For this review, use the dimensioned drawing (mm, ordinates from the lowest corner) and the shaded views. A direction names the side the tool comes from. Coordinates: 2 decimals unless noted, no trailing zeros. Order: outer loops, then holes, each group sorted by start corner. A loop starts at its lowest first (then second) coordinate and runs counter-clockwise, first axis right, second up. Notation, with made-up numbers: M 78.5,56.25 L 127.5,56.25 A17 ccw 127.5,67.25 Z; hole C -5,50.5 d5. An arc over 180 degrees is marked long. Answer in a Markdown table with one row per item.
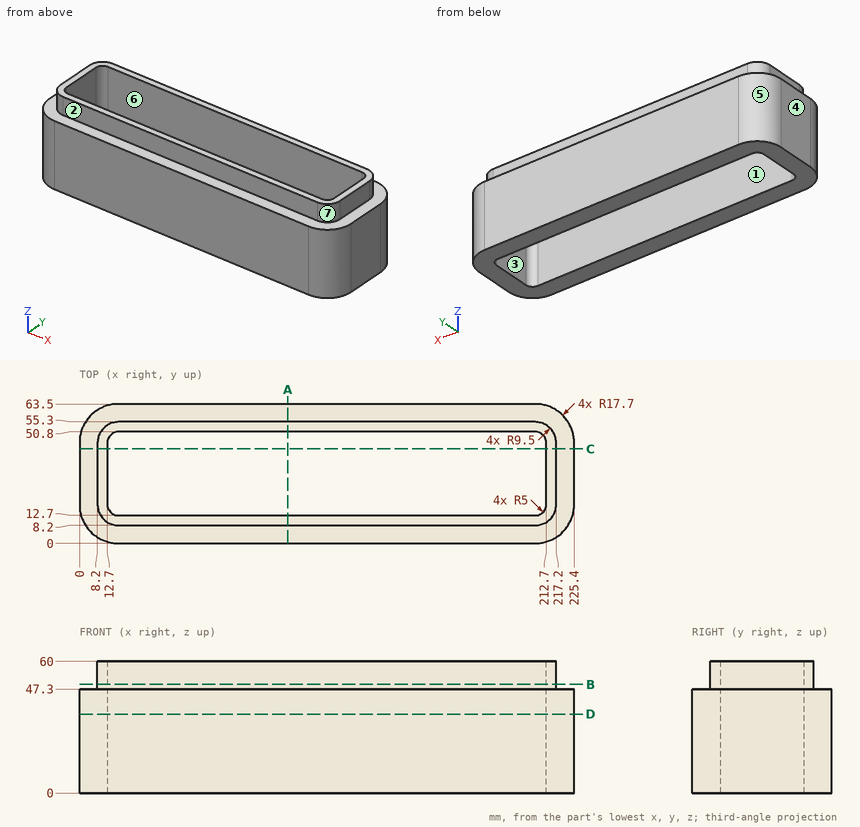
(1) Take a section at D-D (z = 36). Write out the cut boundary in (x, y), then the cut area to 3 significant figures.
Report:
| item | result |
|---|---|
| outline | M 0,17.7 A17.7 ccw 17.7,0 L 207.7,0 A17.7 ccw 225.4,17.7 L 225.4,45.8 A17.7 ccw 207.7,63.5 L 17.7,63.5 A17.7 ccw 0,45.8 Z; hole M 12.7,17.7 A5 ccw 17.7,12.7 L 207.7,12.7 A5 ccw 212.7,17.7 L 212.7,45.8 A5 ccw 207.7,50.8 L 17.7,50.8 A5 ccw 12.7,45.8 Z |
| area | 6,450 mm^2 |
(2) Take a section at B-B (z = 49.5). Write out the cut boundary in (x, y).
Report:
| item | result |
|---|---|
| outline | M 8.2,17.7 A9.5 ccw 17.7,8.2 L 207.7,8.2 A9.5 ccw 217.2,17.7 L 217.2,45.8 A9.5 ccw 207.7,55.3 L 17.7,55.3 A9.5 ccw 8.2,45.8 Z; hole M 12.7,17.7 A5 ccw 17.7,12.7 L 207.7,12.7 A5 ccw 212.7,17.7 L 212.7,45.8 A5 ccw 207.7,50.8 L 17.7,50.8 A5 ccw 12.7,45.8 Z |
(3) Take a section at A-A (x = 95). Write out the cut boundary in (y, z).
Report:
| item | result |
|---|---|
| outline | M 0,0 L 12.7,0 L 12.7,60 L 8.2,60 L 8.2,47.3 L 0,47.3 Z; M 50.8,0 L 63.5,0 L 63.5,47.3 L 55.3,47.3 L 55.3,60 L 50.8,60 Z |
(4) Take a section at C-C (y = 43). Write out the cut boundary in (x, z).
Report:
| item | result |
|---|---|
| outline | M 0,0 L 12.7,0 L 12.7,60 L 8.2,60 L 8.2,47.3 L 0,47.3 Z; M 212.7,0 L 225.4,0 L 225.4,47.3 L 217.2,47.3 L 217.2,60 L 212.7,60 Z |
(5) The part is to be moulded in two halves that separate along X. For the marked faces 1, 2, 3 and 4, say which applies: +X half, -X half, draft (parallel to the pull), parting line (faces both ways), or undercut.
Report:
| item | result |
|---|---|
| face 1 | undercut |
| face 2 | draft |
| face 3 | undercut |
| face 4 | -X half |
(6) Machinability: for the marked faces 5, 6 and 7, which of the approach directions +Z, -Z, +X, -X, +Y, -Y give a long, thin tool a straight path to every point of the face, cutting with its end or side? Answer none if there is none.
Report:
| item | result |
|---|---|
| face 5 | +Z, -Z, -X, +Y |
| face 6 | +Z, -Z |
| face 7 | +Z, +X, -Y |
(7) To check wall thickness, follow line 1 (Y direction, x = 156.5, z = 43); line 2 (X direction, y = 18, z = 6); line 3 (X direction, y = 27.5, z = 50.5). State the ranges of each line that lie inside material, in increasing order. Write a range as [from, to].
Report:
| item | result |
|---|---|
| line 1 | [0, 12.7], [50.8, 63.5] |
| line 2 | [0, 12.7], [212.7, 225.4] |
| line 3 | [8.2, 12.7], [212.7, 217.2] |
(8) Insertion check: P1, Ø10, axis at y = 27, z = 53, coming from the -X side; P2, Ø14, axis at y = 25.5, z = 55.5, coming from the +X side; P3, Ø1.5, axis at x = 153.5, y = 14, coming from the +Z side; P4, Ø12, axis at y = 53.5, z = 50.5, coming from the -X side. Each pin has a flat end and moves straight along its axis. Give the tip position at first contact, or say it passes through.
Report:
| item | result |
|---|---|
| P1 | x = 8.2 |
| P2 | x = 217.2 |
| P3 | through |
| P4 | x = 0.2 |
